Could you check a few things on this model? Use its own coordinates, in mm. A direction names the side the tool comes from. Round coordinates to 2 decimals unless told otherwise and drop trailing zeros. Loops run counter-clockwise (first coordinate to the right, second up) from the corner with the lowest first, then second, coordinate; pieces in that order, holes last. Notation, with made-up numbers: (20, -17) -> (27, -17) arc R10 ccw to (27, 2) -> close; hole circle Ø11 at (47.5, -31.5). An arc over 180 degrees is marked (long way). Put each result on its own line as item: value. Start each with the question number.
1. Imagine slicing it at D-D, the plane x = 5. Please give me the cut outline in (y, z), and give its area (3 significant figures).
2. I need wall thicknesses on line 1 (Z direction, x = 0, y = 16); line 2 (Z direction, x = -1.5, y = 28.5). Which ranges of each line are inside material? Lowest first, please. Write a range as [from, to].
3. If we mould it in two halves opening along Z, with no side actions, what happens to faces 4 (the cylindrical face through (2.95, 23.1, -2.7)), 5 (the flat face through (-8.479, 36.476, -14.735)), 6 (the flat face through (-3, -5, 3))? For each: pulls with the +Z half, pulls with the -Z half, needs draft (parallel to the pull), parting line crosses it, or undercut.
4. I'm going to push flat-ended pins straight in: P1, Ø1.6, axis at x = 5, y = 49, coming from the +Z side; P2, Ø5, axis at x = 2, z = 2, coming from the -Y side; P3, Ø2, axis at y = 48.5, z = 5, coming from the +X side; P4, Ø2, axis at x = 2, z = -1.5, coming from the -Y side. Where does each tip first touch, or does it pass through?
5. Which directions (+Z, -Z, +X, -X, +Y, -Y) give clear straight access to the entire face, cutting with the end or side of a thin tool? Please do faces 1 (the flat face through (-5, -2, 0)), 2 (the flat face through (3, 0, 3)), 3 (the flat face through (-3, 47, -3)).
6. Imagine slicing it at C-C, the plane y = 17.5. Please give me the cut outline in (x, z).
7. Imagine slicing it at B-B, the plane z = 2.5. Please give me the cut outline in (x, y).
8. Imagine slicing it at A-A, the plane x = 1.5. Please give me the cut outline in (y, z), and give its area (3 significant figures).
Autodesk Inventor part; units mm, degrees
ref_plane "Work Plane1" through (0, 23.5, 0) normal (0, 1, 0) x (1, 0, 0)
ref_plane "Work Plane2" through (6, 37, 0) normal (1, 0, 0) x (0, 1, 0)
ref_plane "Work Plane3" through (-6.5, 36.5, 11.2583) normal (-0.5, 0, 0.866) x (0.866, 0, 0.5)
sketch "Sketch1" plane through (0, 0, 0) normal (0, 1, 0) x (-1, 0, 0)
  circle A0 centre (0, 0) radius 4
  circle A1 centre (0, 0) radius 6
  dimension "d0" = 8
  dimension "d1" = 12
extrude "Extrusion1" add sketch "Sketch1" along normal blind 47
sketch "Sketch2" plane through (0, 47, 0) normal (0, 1, 0) x (1, 0, 0)
  circle A0 centre (0, 0) radius 6 construction
  arc A1 (-6, 0) -> (0, -6) centre (0, 0) ccw
  circle A2 centre (0, 0) radius 4 construction
  arc A3 (-4, 0) -> (0, -4) centre (0, 0) ccw
  line L0 (0, -6) -> (0, -4)
  line L1 (-4, 0) -> (-6, 0)
  line L2 (4, 0) -> (6, 0)
  arc A4 (6, 0) -> (0, 6) centre (0, 0) ccw
  arc A5 (4, 0) -> (0, 4) centre (0, 0) ccw
  line L3 (0, 6) -> (0, 4)
  dimension "d6" = 360
extrude "Extrusion2" add sketch "Sketch2" along normal blind 5
ref_plane "Work Plane5" through (0, 37, 0) normal (0, -1, 0) x (1, 0, 0)
ref_plane "Work Plane1" through (0, 23.5, 0) normal (0, 1, 0) x (1, 0, 0)
mirror "Mirror1" about plane through (0, 23.5, 0) normal (0, 1, 0) of "Extrusion2"
sketch "Sketch3" plane through (0, 37, 0) normal (0, -1, 0) x (1, 0, 0)
  arc A0 (-6, 0) -> (0, -6) centre (0, 0) ccw construction
  line L0 (0, -6) -> (0, -4) construction
  arc A1 (-4, 0) -> (0, -4) centre (0, 0) ccw construction
  line L1 (-4, 0) -> (-6, 0) construction
  line L2 (-6, 0) -> (-4, 0) construction
  arc A2 (0, 4) -> (-4, 0) centre (0, 0) ccw construction
  line L3 (0, 4) -> (0, 6) construction
  arc A3 (0, 6) -> (-6, 0) centre (0, 0) ccw construction
  arc A4 (4, 0) -> (0, 4) centre (0, 0) ccw construction
  line L4 (4, 0) -> (6, 0) construction
  arc A5 (6, 0) -> (0, 6) centre (0, 0) ccw construction
  line L5 (0, 6) -> (0, 4) construction
  line L6 (0, -4) -> (0, -6) construction
  arc A6 (0, -6) -> (6, 0) centre (0, 0) ccw construction
  line L7 (6, 0) -> (4, 0) construction
  arc A7 (0, -4) -> (4, 0) centre (0, 0) ccw construction
  line L8 (6, 0) -> (11.7956, 0) construction
  line L9 (0, 0) -> (-6.4031, -11.0905) construction
  line L10 (0, 0) -> (-6.364, 11.0227) construction
  dimension "d10" = 120
  dimension "d11" = 120
ref_plane "Work Plane2" through (6, 37, 0) normal (1, 0, 0) x (0, 1, 0)
sketch "Sketch4" plane through (6, 37, 0) normal (1, 0, 0) x (0, 1, 0)
  line L0 (-42, -6) -> (-42, 0) construction
  circle A0 centre (-0.5, 0) radius 1.75
  point P0 (-37, 0)
  dimension "d12" = 41.5
  dimension "d38" = 3.5
extrude "Extrusion3" add sketch "Sketch4" along normal blind 11 and the other way blind 0.5
pattern_circular "Circular Pattern1" count 3 over 360 about axis through (0, 0, 0) along (0, 1, 0) of "Extrusion3"
thread "Thread1"
thread "Thread2"
thread "Thread3"
ref_plane "Work Plane3" through (-6.5, 36.5, 11.2583) normal (-0.5, 0, 0.866) x (0.866, 0, 0.5)
sketch "Sketch6" plane through (-6.5, 36.5, 11.2583) normal (-0.5, 0, 0.866) x (0.866, 0, 0.5)
  line L0 (0, 0) -> (-3.1225, -1.8028) construction
  line L1 (0, 0) -> (0, 3.8525) construction
  point P0 (0, -36.5)
  point P1 (-1.7321, -1)
  dimension "d27" = 120
ref_plane "Work Plane4" through (-8, 35.5, 10.3923) normal (-0.75, -0.5, -0.433) x (0.5547, -0.8321, 0)
sketch "Sketch7" plane through (-8, 35.5, 10.3923) normal (-0.75, -0.5, -0.433) x (0.5547, -0.8321, 0)
  point P0 (33.9754, -3.723)
  point P1 (0, 0)
hole "Hole1" at (-8, 35.5, 10.3923) direction (0.75, 0.5, 0.433) diameter 1 end through all
pattern_circular "Circular Pattern2" count 3 over 360 about axis through (0, 0, 0) along (0, 1, 0) of "Hole1"
properties part number "ObererRührerHalter"
Entries:
1. outline: (-5, -3.32) -> (52, -3.32) -> (52, 0) -> (47, 0) -> (47, 3.32) -> (0, 3.32) -> (0, 0) -> (-5, 0) -> close
1. area: 345 mm^2
2. line 1: [-6, -4], [4, 6]
2. line 2: [-5.81, -3.71], [3.71, 5.81]
3. face 4: undercut
3. face 5: pulls with the -Z half
3. face 6: needs draft
4. P1: z = 0
4. P2: y = 0
4. P3: x = 0
4. P4: through
5. face 1: -Z, -X, -Y
5. face 2: +Z, +X, -Y
5. face 3: -Z, -X, +Y
6. outline: circle Ø12 at (0, 0); hole circle Ø8 at (0, 0)
7. outline: (-5.45, -5) -> (-3.12, -5) -> (-3.12, 52) -> (-5.45, 52) -> close; (3.12, 0) -> (5.45, 0) -> (5.45, 47) -> (3.12, 47) -> close
8. outline: (-5, -5.81) -> (52, -5.81) -> (52, -3.71) -> (-5, -3.71) -> close; (0, 3.71) -> (47, 3.71) -> (47, 5.81) -> (0, 5.81) -> close
8. area: 219 mm^2
